```python
from build123d import *

# Parameters (mm, degrees)
BOSS_EXTRUDE1_DEPTH = 1.6
SKETCH2_R           = 2.495
BOSS_EXTRUDE2_DEPTH = 0.05
SKETCH3_R           = 1.6
CUT_EXTRUDE1_DEPTH  = 15.58929402
SKETCH4_W           = 7
SKETCH4_H           = 12
BOSS_EXTRUDE3_DEPTH = 4


with BuildPart() as part:
    # Sketch1 → Boss-Extrude1 (new body)
    with BuildSketch(Plane(origin=(0, 0, 0), x_dir=(1, 0, 0), z_dir=(0, 1, 0))):
        with BuildLine():
            Line((7.75, -10.25), (-7.75, -10.25))
            ThreePointArc((-7.75, -10.25), (-9.517766953, -9.517766953), (-10.25, -7.75))
            Line((-10.25, -7.75), (-10.25, 7.75))
            ThreePointArc((-10.25, 7.75), (-9.517766953, 9.517766953), (-7.75, 10.25))
            Line((-7.75, 10.25), (7.75, 10.25))
            ThreePointArc((7.75, 10.25), (9.517766953, 9.517766953), (10.25, 7.75))
            Line((10.25, 7.75), (10.25, -7.75))
            ThreePointArc((10.25, -7.75), (9.517766953, -9.517766953), (7.75, -10.25))
        make_face()
    extrude(amount=BOSS_EXTRUDE1_DEPTH)

    # Sketch2 → Boss-Extrude2 (add)
    with BuildSketch(Plane(origin=(0, 1.6, 0), x_dir=(1, 0, 0), z_dir=(0, 1, 0))):
        with Locations(Location((-7.75, 7.75, 0), (0, 0, 90))):
            Circle(SKETCH2_R)
        with Locations(Location((7.75, 7.75, 0), (0, 0, 90))):
            Circle(SKETCH2_R)
        with Locations(Location((7.75, -7.75, 0), (0, 0, 90))):
            Circle(SKETCH2_R)
        with Locations(Location((-7.75, -7.75, 0), (0, 0, 90))):
            Circle(SKETCH2_R)
    extrude(amount=BOSS_EXTRUDE2_DEPTH)

    # Sketch3 → Cut-Extrude1 (cut, through all)
    with BuildSketch(Plane(origin=(0, 1.65, 0), x_dir=(1, 0, 0), z_dir=(0, 1, 0))):
        with Locations(Location((-7.75, 7.75, 0), (0, 0, 270))):
            Circle(SKETCH3_R)
        with Locations(Location((7.75, 7.75, 0), (0, 0, 270))):
            Circle(SKETCH3_R)
        with Locations(Location((7.75, -7.75, 0), (0, 0, 270))):
            Circle(SKETCH3_R)
        with Locations(Location((-7.75, -7.75, 0), (0, 0, 270))):
            Circle(SKETCH3_R)
    extrude(amount=-CUT_EXTRUDE1_DEPTH, mode=Mode.SUBTRACT)

    # Sketch4 → Boss-Extrude3 (add)
    with BuildSketch(Plane(origin=(0, 1.6, 0), x_dir=(1, 0, 0), z_dir=(0, 1, 0))):
        with Locations((-6.7, 0)):
            Rectangle(SKETCH4_W, SKETCH4_H)
    extrude(amount=BOSS_EXTRUDE3_DEPTH)


solid = part.part
```
Read the model definition and answer for the solid it produces. Units are mm, in the model's axes. A direction names the side the tool comes from. Give positions to 0.01 mm unless a question says otherwise; leave off trailing zeros. Loops run counter-clockwise (first coordinate to the right, second up) from the corner with the lowest first, then second, coordinate; pieces in that order, holes last.
Item 1: The part is cut by section C-C (x = -2.25). Write down the section's boundary in (y, z), and give its area (3 significant figures).
Item 2: The mould has two halves that part along Z. Classify faces 1 (the cylindrical face through (6.19, 0.84, -8.1)), 2 (the cylindrical face through (9.537, 0.789, 9.498)), 3 (the flat face through (-10.25, 1, 0)): released by +Z, released by -Z, zero draft, split by the parting line, or undercut.
Item 3: Find the intervals of material crossed by line 1 along X through (y, z) = (1.2, -7.75); line 2 along Y through (x, z) = (-0.5, -7.25); line 3 along Z through (x, y) = (-3.75, 4.7), in increasing order.
Item 4: Each of these flat-tipped pins is pushed along its axis until it touches: pin 1 Ø5.5 at (x, z) = (7, -7) entering from +Y; pin 2 Ø12 at (x, z) = (5.5, -1.5) entering from -Y; pin 3 Ø3 at (x, z) = (2, 4) entering from +Y; pin 4 Ø1.2 at (y, z) = (3, -1.5) entering from +X. Where does it stop, or does it pass through?
Item 5: The part is cut by section A-A (z = -8.5). Give the number of separate pieces and of enclosed holes in the cut face, and give its area (3 significant figures).
Item 6: The part is cut by section B-B (z = 3). Write down the section's boundary in (x, y).
Item 7: The part is cut by section D-D (y = 4.95). Write down the section's boundary in (x, z).
Item 8: For faces 4 (the flat face through (2, 1.6, 0)), 5 (the cylindrical face through (-9.537, 0.789, -9.498)), determine the directions among +Z, -Z, +X, -X, +Y, -Y from which every point of the face is accessible in a straight line to the end or side of a thin tool.
Taken from the geometry:
1. outline: (0, -10.25) - (1.6, -10.25) - (1.6, 10.25) - (0, 10.25) - close
1. area: 32.8 mm2
2. face 1: undercut
2. face 2: released by +Z
2. face 3: zero draft
3. line 1: x = -10.25 to -9.35, -6.15 to 6.15, 9.35 to 10.25
3. line 2: y = 0 to 1.6
3. line 3: z = -6 to 6
4. pin 1: stops at y = 1.65
4. pin 2: stops at y = 0
4. pin 3: stops at y = 1.6
4. pin 4: stops at x = -3.2
5. separate pieces: 3
5. enclosed holes: 0
5. area: 23.6 mm2
6. outline: (-10.25, 0) - (10.25, 0) - (10.25, 1.6) - (-3.2, 1.6) - (-3.2, 5.6) - (-10.2, 5.6) - (-10.2, 1.6) - (-10.25, 1.6) - close
7. outline: (-10.2, -6) - (-3.2, -6) - (-3.2, 6) - (-10.2, 6) - close
8. face 4: +Y
8. face 5: -Z, -X, +Y, -Y
